Geometry: final body of the model. Coordinates: model frame, mm. A direction names the side the tool comes from. Give positions to 0.01 mm unless a question says otherwise; leave off trailing zeros. Write each loop counter-clockwise with the first axis right and the second up, starting at its lowest first coordinate (ties: lowest second). Pieces come first, ordered by that corner, then holes. Notation, with made-up numbers: (21.25, -36.75) -> (80.25, -36.75) arc R21 cw to (80.25, -24.75) -> close; hole circle Ø4 at (59, 23). An arc over 180 degrees is marked (long way). Answer as a JSON object with one key per item and string values. Group by question number.
(1) Section query B-B on z = 0. Output: boundary loops of the cut face in (x, y), plus the area to 4 significant figures.
(2) Section query A-A on x = 0. Output: boundary loops of the cut face in (y, z).
(3) Set-up query: faces 1 (the face through (4.903, -12.325, 24.514)), 2 (the face through (-21.105, -12.325, -17.56)), 3 (the face through (27.412, -12.325, 2.493)). Return all of +Z, -Z, +X, -X, +Y, -Y with unobstructed straight access to the full face (end or side cutting, diameter ignored); none if empty.
(4) Material intervals for probe 1 along Z at (x, y) = (0, -9.5); probe 2 along X at (y, z) = (-8, -26); probe 3 along Z at (x, y) = (-20, -21), sorted ascending.
(5) Draft query along Z for faces 4 (the face through (12.05, -12.32, 6.66)), 5 (the face through (24.514, -12.325, -4.903)), 6 (the face through (17.62, -12.325, 21.146)), 7 (the face through (-17.62, -12.325, -21.146)). Return one class per face: +Z half, -Z half, draft (parallel to the pull), parting line (faces both ways), or undercut.
(6) Contact query for flat-ended pins moving along their axis: pin 1 Ø8 at (x, y) = (18, -16.5) entering from +Z; pin 2 Ø4 at (y, z) = (-17, 17.5) entering from +X; pin 3 Ø2 at (y, z) = (-19.5, 23) entering from +X; pin 4 Ø3.5 at (x, z) = (0, 15) entering from +Y. Output: stop coordinate, or through.
(7) Section query C-C on y = -12.5. State how many separate pieces and enclosed holes the cut face has, plus the area to 3 significant figures.
from build123d import *

# Parameters (mm, degrees)
F0_R     = 3
F0_R_2   = 7.5
F1_DEPTH = 25


with BuildPart() as f1:
    # F0 (on Front) → F1 (new body)
    with BuildSketch(Plane.XZ):
        with BuildLine():
            ThreePointArc((24.819347, -3), (24.954796, -1.502717), (25, 0))
            ThreePointArc((25, 0), (24.954796, 1.502717), (24.819347, 3))
            ThreePointArc((24.819347, 3), (24.519632, 4.877258), (24.078137, 6.726314))
            ThreePointArc((24.078137, 6.726314), (23.096988, 9.567086), (21.782037, 12.269592))
            ThreePointArc((21.782037, 12.269592), (20.78674, 13.889256), (19.671249, 15.428608))
            ThreePointArc((19.671249, 15.428608), (17.67767, 17.67767), (15.428608, 19.671249))
            ThreePointArc((15.428608, 19.671249), (13.889256, 20.78674), (12.269592, 21.782037))
            ThreePointArc((12.269592, 21.782037), (9.567086, 23.096988), (6.726314, 24.078137))
            ThreePointArc((6.726314, 24.078137), (4.877258, 24.519632), (3, 24.819347))
            ThreePointArc((3, 24.819347), (0, 25), (-3, 24.819347))
            ThreePointArc((-3, 24.819347), (-4.877258, 24.519632), (-6.726314, 24.078137))
            ThreePointArc((-6.726314, 24.078137), (-9.567086, 23.096988), (-12.269592, 21.782037))
            ThreePointArc((-12.269592, 21.782037), (-13.889256, 20.78674), (-15.428608, 19.671249))
            ThreePointArc((-15.428608, 19.671249), (-17.67767, 17.67767), (-19.671249, 15.428608))
            ThreePointArc((-19.671249, 15.428608), (-20.78674, 13.889256), (-21.782037, 12.269592))
            ThreePointArc((-21.782037, 12.269592), (-23.096988, 9.567086), (-24.078137, 6.726314))
            ThreePointArc((-24.078137, 6.726314), (-24.519632, 4.877258), (-24.819347, 3))
            ThreePointArc((-24.819347, 3), (-25, 0), (-24.819347, -3))
            ThreePointArc((-24.819347, -3), (-24.519632, -4.877258), (-24.078137, -6.726314))
            ThreePointArc((-24.078137, -6.726314), (-23.096988, -9.567086), (-21.782037, -12.269592))
            ThreePointArc((-21.782037, -12.269592), (-20.78674, -13.889256), (-19.671249, -15.428608))
            ThreePointArc((-19.671249, -15.428608), (-17.67767, -17.67767), (-15.428608, -19.671249))
            ThreePointArc((-15.428608, -19.671249), (-13.889256, -20.78674), (-12.269592, -21.782037))
            ThreePointArc((-12.269592, -21.782037), (-9.567086, -23.096988), (-6.726314, -24.078137))
            ThreePointArc((-6.726314, -24.078137), (-4.877258, -24.519632), (-3, -24.819347))
            ThreePointArc((-3, -24.819347), (0, -25), (3, -24.819347))
            ThreePointArc((3, -24.819347), (4.877258, -24.519632), (6.726314, -24.078137))
            ThreePointArc((6.726314, -24.078137), (9.567086, -23.096988), (12.269592, -21.782037))
            ThreePointArc((12.269592, -21.782037), (13.889256, -20.78674), (15.428608, -19.671249))
            ThreePointArc((15.428608, -19.671249), (17.67767, -17.67767), (19.671249, -15.428608))
            ThreePointArc((19.671249, -15.428608), (20.78674, -13.889256), (21.782037, -12.269592))
            ThreePointArc((21.782037, -12.269592), (23.096988, -9.567086), (24.078137, -6.726314))
            ThreePointArc((24.078137, -6.726314), (24.519632, -4.877258), (24.819347, -3))
        make_face()
        with Locations((-8.816779, -12.135255)):
            Circle(F0_R, mode=Mode.SUBTRACT)
        with Locations((8.816779, -12.135255)):
            Circle(F0_R, mode=Mode.SUBTRACT)
        with Locations((-14.265848, 4.635255)):
            Circle(F0_R, mode=Mode.SUBTRACT)
        Circle(F0_R_2, mode=Mode.SUBTRACT)
        with Locations((14.265848, 4.635255)):
            Circle(F0_R, mode=Mode.SUBTRACT)
        with Locations((0, 15)):
            Circle(F0_R, mode=Mode.SUBTRACT)
        with BuildLine():
            ThreePointArc((24.819347, 3), (24.954796, 1.502717), (25, 0))
            ThreePointArc((25, 0), (24.954796, -1.502717), (24.819347, -3))
            Line((24.819347, -3), (29.933259, -2))
            ThreePointArc((29.933259, -2), (30, 0), (29.933259, 2))
            Line((29.933259, 2), (24.819347, 3))
        make_face()
        with BuildLine():
            ThreePointArc((21.782037, 12.269592), (23.096988, 9.567086), (24.078137, 6.726314))
            Line((24.078137, 6.726314), (28.420092, 9.607203))
            ThreePointArc((28.420092, 9.607203), (27.716386, 11.480503), (26.889359, 13.302721))
            Line((26.889359, 13.302721), (21.782037, 12.269592))
        make_face()
        with BuildLine():
            Line((28.420092, -9.607203), (24.078137, -6.726314))
            ThreePointArc((24.078137, -6.726314), (23.096988, -9.567086), (21.782037, -12.269592))
            Line((21.782037, -12.269592), (26.889359, -13.302721))
            ThreePointArc((26.889359, -13.302721), (27.716386, -11.480503), (28.420092, -9.607203))
        make_face()
        with BuildLine():
            ThreePointArc((15.428608, 19.671249), (17.67767, 17.67767), (19.671249, 15.428608))
            Line((19.671249, 15.428608), (22.580224, 19.751797))
            ThreePointArc((22.580224, 19.751797), (21.213203, 21.213203), (19.751797, 22.580224))
            Line((19.751797, 22.580224), (15.428608, 19.671249))
        make_face()
        with BuildLine():
            Line((22.580224, -19.751797), (19.671249, -15.428608))
            ThreePointArc((19.671249, -15.428608), (17.67767, -17.67767), (15.428608, -19.671249))
            Line((15.428608, -19.671249), (19.751797, -22.580224))
            ThreePointArc((19.751797, -22.580224), (21.213203, -21.213203), (22.580224, -19.751797))
        make_face()
        with BuildLine():
            ThreePointArc((6.726314, 24.078137), (9.567086, 23.096988), (12.269592, 21.782037))
            Line((12.269592, 21.782037), (13.302721, 26.889359))
            ThreePointArc((13.302721, 26.889359), (11.480503, 27.716386), (9.607203, 28.420092))
            Line((9.607203, 28.420092), (6.726314, 24.078137))
        make_face()
        with BuildLine():
            Line((13.302721, -26.889359), (12.269592, -21.782037))
            ThreePointArc((12.269592, -21.782037), (9.567086, -23.096988), (6.726314, -24.078137))
            Line((6.726314, -24.078137), (9.607203, -28.420092))
            ThreePointArc((9.607203, -28.420092), (11.480503, -27.716386), (13.302721, -26.889359))
        make_face()
        with BuildLine():
            ThreePointArc((-3, 24.819347), (0, 25), (3, 24.819347))
            Line((3, 24.819347), (2, 29.933259))
            ThreePointArc((2, 29.933259), (0, 30), (-2, 29.933259))
            Line((-2, 29.933259), (-3, 24.819347))
        make_face()
        with BuildLine():
            Line((2, -29.933259), (3, -24.819347))
            ThreePointArc((3, -24.819347), (0, -25), (-3, -24.819347))
            Line((-3, -24.819347), (-2, -29.933259))
            ThreePointArc((-2, -29.933259), (0, -30), (2, -29.933259))
        make_face()
        with BuildLine():
            ThreePointArc((-12.269592, 21.782037), (-9.567086, 23.096988), (-6.726314, 24.078137))
            Line((-6.726314, 24.078137), (-9.607203, 28.420092))
            ThreePointArc((-9.607203, 28.420092), (-11.480503, 27.716386), (-13.302721, 26.889359))
            Line((-13.302721, 26.889359), (-12.269592, 21.782037))
        make_face()
        with BuildLine():
            Line((-9.607203, -28.420092), (-6.726314, -24.078137))
            ThreePointArc((-6.726314, -24.078137), (-9.567086, -23.096988), (-12.269592, -21.782037))
            Line((-12.269592, -21.782037), (-13.302721, -26.889359))
            ThreePointArc((-13.302721, -26.889359), (-11.480503, -27.716386), (-9.607203, -28.420092))
        make_face()
        with BuildLine():
            ThreePointArc((-19.671249, 15.428608), (-17.67767, 17.67767), (-15.428608, 19.671249))
            Line((-15.428608, 19.671249), (-19.751797, 22.580224))
            ThreePointArc((-19.751797, 22.580224), (-21.213203, 21.213203), (-22.580224, 19.751797))
            Line((-22.580224, 19.751797), (-19.671249, 15.428608))
        make_face()
        with BuildLine():
            Line((-19.751797, -22.580224), (-15.428608, -19.671249))
            ThreePointArc((-15.428608, -19.671249), (-17.67767, -17.67767), (-19.671249, -15.428608))
            Line((-19.671249, -15.428608), (-22.580224, -19.751797))
            ThreePointArc((-22.580224, -19.751797), (-21.213203, -21.213203), (-19.751797, -22.580224))
        make_face()
        with BuildLine():
            ThreePointArc((-24.078137, 6.726314), (-23.096988, 9.567086), (-21.782037, 12.269592))
            Line((-21.782037, 12.269592), (-26.889359, 13.302721))
            ThreePointArc((-26.889359, 13.302721), (-27.716386, 11.480503), (-28.420092, 9.607203))
            Line((-28.420092, 9.607203), (-24.078137, 6.726314))
        make_face()
        with BuildLine():
            Line((-26.889359, -13.302721), (-21.782037, -12.269592))
            ThreePointArc((-21.782037, -12.269592), (-23.096988, -9.567086), (-24.078137, -6.726314))
            Line((-24.078137, -6.726314), (-28.420092, -9.607203))
            ThreePointArc((-28.420092, -9.607203), (-27.716386, -11.480503), (-26.889359, -13.302721))
        make_face()
        with BuildLine():
            ThreePointArc((-24.819347, -3), (-25, 0), (-24.819347, 3))
            Line((-24.819347, 3), (-29.933259, 2))
            ThreePointArc((-29.933259, 2), (-30, 0), (-29.933259, -2))
            Line((-29.933259, -2), (-24.819347, -3))
        make_face()
    extrude(amount=F1_DEPTH)


solid = f1.part
Answer list:
{
 "1": {"outline": "(-30, -25) -> (-7.5, -25) -> (-7.5, 0) -> (-30, 0) -> close; (7.5, -25) -> (30, -25) -> (30, 0) -> (7.5, 0) -> close", "area": "1,125 mm2"},
 "2": {"outline": "(-25, -30) -> (0, -30) -> (0, -7.5) -> (-25, -7.5) -> close; (-25, 7.5) -> (0, 7.5) -> (0, 12) -> (-25, 12) -> close; (-25, 18) -> (0, 18) -> (0, 30) -> (-25, 30) -> close"},
 "3": {"face 1": "+Z, +Y, -Y", "face 2": "-X, +Y, -Y", "face 3": "+X, +Y, -Y"},
 "4": {"probe 1": "-30 to -7.5, 7.5 to 12, 18 to 30", "probe 2": "-13.12 to -8, -2.77 to 2.77, 8 to 13.12", "probe 3": "-22.36 to -15.92, -15 to 15, 15.92 to 22.36"},
 "5": {"face 4": "undercut", "face 5": "undercut", "face 6": "+Z half", "face 7": "-Z half"},
 "6": {"pin 1": "z = 22.58", "pin 2": "x = 22.41", "pin 3": "x = 20.4", "pin 4": "through"},
 "7": {"separate pieces": "1", "enclosed holes": "6", "area": "2,050 mm2"}
}
